Here's how the part is built. I have some questions about the finished solid (model axes, mm). A direction names the side the tool comes from. Round coordinates to 2 decimals unless told otherwise and drop trailing zeros. Write each loop counter-clockwise with the first axis right and the second up, starting at its lowest first coordinate (ties: lowest second). Pieces come first, ordered by that corner, then holes. Notation, with made-up numbers: (68.5, 38.25) - (97.5, 38.25) arc R19 cw to (97.5, 60.25) - close; hole circle Ø9 at (41.5, -31.5). An arc over 180 degrees is marked (long way). Return JSON: item names as keys, results as strings. Group by question number.
```python
from build123d import *

# Parameters (mm, degrees)
TOP_EDGE_OUTLINE_W  = 86.5
TOP_EDGE_OUTLINE_H  = 39.5
TOP_EDGE_DEPTH      = 3
TOP_EDGE_DRAFT      = 45
SKETCH13_W          = 72
SKETCH13_H          = 25
DISPLAY_HOLE_DEPTH  = 6
SKETCH14_W          = 92.5
SKETCH14_H          = 45.5
SKETCH14_W_2        = 89.5
SKETCH14_H_2        = 42.5
BOSS_EXTRUDE5_DEPTH = 5
SKETCH15_W          = 128.5
SKETCH15_H          = 45.5
SKETCH15_W_2        = 89.5
SKETCH15_H_2        = 42.5
BOSS_EXTRUDE6_DEPTH = 2
SKETCH16_W          = 128.5
SKETCH16_H          = 45.5
SKETCH16_W_2        = 125.5
SKETCH16_H_2        = 42.5
BOSS_EXTRUDE7_DEPTH = 37
LOFT2_OUTLINE_W     = 33
LOFT2_OUTLINE_H     = 42.5
LOFT2_DEPTH         = 1.5
LOFT2_DRAFT         = 45
SKETCH19_R          = 2.75
SKETCH19_R_2        = 2
BOSS_EXTRUDE8_DEPTH = 1
CUT_EXTRUDE3_START  = -11
SKETCH20_R          = 2
CUT_EXTRUDE3_DEPTH  = 11
SKETCH21_W          = 12
SKETCH21_H          = 8
CUT_EXTRUDE4_DEPTH  = 11
SKETCH22_W          = 4
SKETCH22_H          = 15
BOSS_EXTRUDE9_DEPTH = 3
SKETCH24_W          = 42.5
SKETCH24_H          = 37
CUT_EXTRUDE5_DEPTH  = 17
SKETCH26_W          = 144.369132995
SKETCH26_H          = 91.038744315
CUT_EXTRUDE6_DEPTH  = 87
SKETCH27_W          = 64.71229982
SKETCH27_H          = 55.593249081
CUT_EXTRUDE7_DEPTH  = 148
SKETCH29_W          = 36
SKETCH29_H          = 45.5
SKETCH29_W_2        = 32.7
SKETCH29_H_2        = 42.2
CUT_EXTRUDE8_DEPTH  = 2


# Read off the part's stored shape, not the designer's step: Top Edge, Loft2
with BuildPart() as part:
    # Top Edge outline → Top Edge (with draft: the straight prism first)
    with BuildSketch(Plane(origin=(0, 0, 0), x_dir=(1, 0, 0), z_dir=(0, 1, 0))):
        with Locations((0.25, -0.25)):
            Rectangle(TOP_EDGE_OUTLINE_W, TOP_EDGE_OUTLINE_H)
    extrude(amount=-TOP_EDGE_DEPTH)
    # Top Edge: the draft: its side faces are tilted about the plane it starts from
    top_edge_sides = [part.faces().sort_by_distance(p)[0] for p in [
        (-43, -1.5, 0.25),
        (0.25, -1.5, 20),
        (43.5, -1.5, 0.25),
        (0.25, -1.5, -19.5),
    ]]
    draft(top_edge_sides, Plane(origin=(0, 0, 0), x_dir=(1, 0, 0), z_dir=(0, 1, 0)), TOP_EDGE_DRAFT)

    # Sketch13 → Display Hole (cut)
    with BuildSketch(Plane(origin=(0, 0, 0), x_dir=(1, 0, 0), z_dir=(0, 1, 0))):
        Rectangle(SKETCH13_W, SKETCH13_H)
    extrude(amount=-DISPLAY_HOLE_DEPTH, mode=Mode.SUBTRACT)

    # Sketch14 → Boss-Extrude5 (add)
    with BuildSketch(Plane.XZ.offset(3)):
        with Locations((0.25, 0.25)):
            Rectangle(SKETCH14_W, SKETCH14_H)
        with Locations((0.25, 0.25)):
            Rectangle(SKETCH14_W_2, SKETCH14_H_2, mode=Mode.SUBTRACT)
    extrude(amount=BOSS_EXTRUDE5_DEPTH)

    # Sketch15 → Boss-Extrude6 (add)
    with BuildSketch(Plane.XZ.offset(8)):
        with Locations((18.25, 0.25)):
            Rectangle(SKETCH15_W, SKETCH15_H)
        with Locations((0.25, 0.25)):
            Rectangle(SKETCH15_W_2, SKETCH15_H_2, mode=Mode.SUBTRACT)
    extrude(amount=BOSS_EXTRUDE6_DEPTH)

    # Sketch16 → Boss-Extrude7 (add)
    with BuildSketch(Plane.XZ.offset(10)):
        with Locations((18.25, 0.25)):
            Rectangle(SKETCH16_W, SKETCH16_H)
        with Locations((18.25, 0.25)):
            Rectangle(SKETCH16_W_2, SKETCH16_H_2, mode=Mode.SUBTRACT)
    extrude(amount=BOSS_EXTRUDE7_DEPTH)


with BuildPart() as loft2_tool:
    # Loft2 outline → Loft2 (with draft: the straight prism first)
    with BuildSketch(Plane(origin=(0, -6.5, 0), x_dir=(1, 0, 0), z_dir=(0, 1, 0))):
        with Locations((64.5, -0.25)):
            Rectangle(LOFT2_OUTLINE_W, LOFT2_OUTLINE_H)
    extrude(amount=-LOFT2_DEPTH)
    # Loft2: the draft: its side faces are tilted about the plane it starts from
    loft2_sides = [loft2_tool.faces().sort_by_distance(p)[0] for p in [
        (81, -7.25, 0.25),
        (64.5, -7.25, -21),
        (48, -7.25, 0.25),
        (64.5, -7.25, 21.5),
    ]]
    draft(loft2_sides, Plane(origin=(0, -6.5, 0), x_dir=(1, 0, 0), z_dir=(0, 1, 0)), LOFT2_DRAFT)


with BuildPart() as part_1:
    add(part.part)

    # Loft2: add loft2_tool
    add(loft2_tool.part)

    # Sketch19 → Boss-Extrude8 (add)
    with BuildSketch(Plane(origin=(0, -6.5, 0), x_dir=(1, 0, 0), z_dir=(0, 1, 0))):
        with Locations(Location((64.5, 3, 0), (0, 0, 270))):
            Circle(SKETCH19_R)
        with Locations(Location((64.5, 3, 0), (0, 0, 270))):
            Circle(SKETCH19_R_2, mode=Mode.SUBTRACT)
    extrude(amount=BOSS_EXTRUDE8_DEPTH)

    # Sketch20 → Cut-Extrude3 (cut)
    with BuildSketch(Plane(origin=(0, -6.5, 0), x_dir=(1, 0, 0), z_dir=(0, 1, 0)).offset(CUT_EXTRUDE3_START)):
        with Locations(Location((64.5, 3, 0), (0, 0, 90))):
            Circle(SKETCH20_R)
    extrude(amount=CUT_EXTRUDE3_DEPTH, mode=Mode.SUBTRACT)

    # Sketch21 → Cut-Extrude4 (cut)
    with BuildSketch(Plane(origin=(82.5, 0, 0), x_dir=(0, 0, -1), z_dir=(1, 0, 0))):
        with Locations((0, -43)):
            Rectangle(SKETCH21_W, SKETCH21_H)
    extrude(amount=-CUT_EXTRUDE4_DEPTH, mode=Mode.SUBTRACT)

    # Sketch22 → Boss-Extrude9 (add)
    with BuildSketch(Plane.XZ.offset(3)):
        with Locations((-38, 0)):
            Rectangle(SKETCH22_W, SKETCH22_H)
    extrude(amount=BOSS_EXTRUDE9_DEPTH)

    # Sketch24 → Cut-Extrude5 (cut)
    with BuildSketch(Plane.ZY.offset(-81)):
        with Locations((0.25, -28.5)):
            Rectangle(SKETCH24_W, SKETCH24_H)
    extrude(amount=-CUT_EXTRUDE5_DEPTH, mode=Mode.SUBTRACT)

    # Sketch26 → Cut-Extrude6 (cut)
    with BuildSketch(Plane.XZ.offset(10)):
        with Locations((18.609127197, -2.802581171)):
            Rectangle(SKETCH26_W, SKETCH26_H)
    extrude(amount=CUT_EXTRUDE6_DEPTH, mode=Mode.SUBTRACT)

    # Sketch27 → Cut-Extrude7 (cut)
    with BuildSketch(Plane(origin=(46.5, 0, 0), x_dir=(0, 0, -1), z_dir=(1, 0, 0))):
        with Locations((3.100976476, -7.362126245)):
            Rectangle(SKETCH27_W, SKETCH27_H)
    extrude(amount=-CUT_EXTRUDE7_DEPTH, mode=Mode.SUBTRACT)

    # Sketch29 → Cut-Extrude8 (cut)
    with BuildSketch(Plane.XZ.offset(10)):
        with Locations((64.5, 0.25)):
            Rectangle(SKETCH29_W, SKETCH29_H)
        with Locations((64.5, 0.25)):
            Rectangle(SKETCH29_W_2, SKETCH29_H_2, mode=Mode.SUBTRACT)
    extrude(amount=-CUT_EXTRUDE8_DEPTH, mode=Mode.SUBTRACT)


solid = part_1.part
```
1) Imagine slicing it at D-D (z = 16). Please give me the cut outline in (x, y).
2) Imagine slicing it at A-A (z = -3). Please give me the cut outline in (x, y).
3) If we mould it in two halves opening along Z, with no side actions, what happens to faces 1 (the flat face through (64, -6.5, 0)), 2 (the flat face through (64.2, -7.2, -21.7)), 3 (the cylindrical face through (62.504, -7.781, -3.132))? For each: released by +Z, released by -Z, zero draft, split by the parting line, or undercut.
4) I need wall thicknesses on line 1 along X through (y, z) = (-8.7, -3); line 2 along Y through (x, z) = (70, -1.5); line 3 along Z through (x, y) = (64.5, -8.4). Which ranges of each line are inside material? Lowest first, please.
5) Will these pins go through, and if not, where does the flat tip stop? pin 1 Ø2 at (x, y) = (57, -9.5) entering from -Z; pin 2 Ø0.6 at (x, y) = (59, -9.5) entering from +Z; pin 3 Ø1.5 at (y, z) = (-8, -12) entering from +X.
6) Imagine slicing it at C-C (x = 64.5). Please give me the cut outline in (y, z), plus the area to 3 significant figures.
7) Imagine slicing it at B-B (y = -9.25). Please give me the cut outline in (x, z), plus the area to 3 significant figures.
8) For faces 4 (the flat face through (48.15, -9, 0)), 5 (the flat face through (80.85, -9, 0)), 6 (the flat face through (64, -9, 21.35)), 7 (the cylindrical face through (67.227, -6.007, -3.358)), which set-ups out of +Z, -Z, +X, -X, +Y, -Y let a thin tool reach every point of the face, with its end or its side?
Results found:
{
 "1": {"outline": "(46.5, -8) - (48.15, -8) - (48.15, -10) - (80.85, -10) - (80.85, -8) - (82.5, -8) - (81, -6.5) - (48, -6.5) - close"},
 "2": {"outline": "(46.5, -8) - (48.15, -8) - (48.15, -10) - (62.5, -10) - (62.5, -5.5) - (61.75, -5.5) - (61.75, -6.5) - (48, -6.5) - close; (66.5, -10) - (80.85, -10) - (80.85, -8) - (82.5, -8) - (81, -6.5) - (67.25, -6.5) - (67.25, -5.5) - (66.5, -5.5) - close"},
 "3": {"face 1": "zero draft", "face 2": "released by -Z", "face 3": "undercut"},
 "4": {"line 1": "x = 48.15 to 62.5, 66.5 to 80.85", "line 2": "y = -10 to -6.5", "line 3": "z = -20.85 to -5, -1 to 21.35"},
 "5": {"pin 1": "stops at z = -20.85", "pin 2": "stops at z = 21.35", "pin 3": "stops at x = 82.5"},
 "6": {"outline": "(-10, -20.85) - (-8, -20.85) - (-8, -22.5) - (-6.5, -21) - (-6.5, -5.75) - (-5.5, -5.75) - (-5.5, -5) - (-10, -5) - close; (-10, -1) - (-5.5, -1) - (-5.5, -0.25) - (-6.5, -0.25) - (-6.5, 21.5) - (-8, 23) - (-8, 21.35) - (-10, 21.35) - close", "area": "138 mm²"},
 "7": {"outline": "(48.15, -20.85) - (80.85, -20.85) - (80.85, 21.35) - (48.15, 21.35) - close; hole circle Ø4 at (64.5, -3)", "area": "1,370 mm²"},
 "8": {"face 4": "+Z, -Z, -X, -Y", "face 5": "+Z, -Z, +X, -Y", "face 6": "+Z, +X, -X, -Y", "face 7": "+Y"}
}
